For this review, take the finished solid that the model builds, in its own axes (mm). Give positions to 0.01 mm unless a question says otherwise; leave off trailing zeros. Write each loop counter-clockwise with the first axis right and the second up, starting at its lowest first coordinate (ties: lowest second). Pieces come first, ordered by that corner, then holes.
Q1. We need section A-A (z = 0). Write out the cut boundary in (x, y) (3 decimals).
Q2. Insertion check: P1, Ø8.5, axis at x = -29.48, z = 29.48, coming from the -Y side. The pin has a flat end and moves straight along its axis. Give the tip position at first contact, or say it passes through.
Q3. Mouldability with a two-part tool opening along Z and no side actions: class faces 1 (the cylindrical face through (-32.001, 87.072, 31.413)), 2 (the cylindrical face through (-26.454, 87.072, -30.436)), 3 (the flat face through (-35.687, 87, 0)), 4 (the flat face through (0, 87, 35.687)) as released by +Z, released by -Z, zero draft, split by the parting line, or undercut.
Q4. We need section C-C (y = 88.1). Write out the cut boundary in (x, z) (3 decimals), then the cut area to 3 significant figures.
Q5. We need section D-D (x = 29). Write out the cut boundary in (y, z).
Q6. For line 1 (X direction, y = 86.4, z = 31); line 2 (Z direction, x = 0, y = 86.75) (3 decimals), list the stretches that pass through material, from the lowest coordinate up.
Q7. We need section B-B (x = 0). Write out the cut boundary in (y, z) (3 decimals), then the cut area to 3 significant figures.
```python
from build123d import *

# Parameters (mm, degrees)
SKETCH3_W            = 71.374
SKETCH3_H            = 71.374
BOSS_EXTRUDE1_DEPTH  = 88.9508
SHELL1_T             = 5.08
CUT_EXTRUDE1_REACH   = 7.08
SKETCH4_R            = 8.255
SKETCH15_OUTSIDE_W   = 100.282
SKETCH15_OUTSIDE_H   = 117.859
SKETCH15_OUTSIDE_W_2 = 71.374
SKETCH15_OUTSIDE_H_2 = 3.81
CUT_EXTRUDE14_DEPTH  = 72.374
CUT_EXTRUDE15_START  = 88.9508
SKETCH20_R           = 3.175
CUT_EXTRUDE15_DEPTH  = 89.9508
SKETCH6_W            = 71.374
SKETCH6_H            = 5.08
CUT_EXTRUDE3_DEPTH   = 5.08


with BuildPart() as part:
    # Sketch3 → Boss-Extrude1 (new body)
    with BuildSketch(Plane(origin=(0, 0, 0), x_dir=(1, 0, 0), z_dir=(0, 1, 0))):
        Rectangle(SKETCH3_W, SKETCH3_H)
    extrude(amount=BOSS_EXTRUDE1_DEPTH)

    # Shell1 (no face opened: a closed hollow body)
    add(offset(amount=-SHELL1_T, mode=Mode.PRIVATE), mode=Mode.SUBTRACT)

    # Sketch4 → Cut-Extrude1 (cut, up to next)
    with BuildSketch(Plane(origin=(0, 83.8708, 0), x_dir=(-1, 0, 0), z_dir=(0, -1, 0)), mode=Mode.PRIVATE) as cut_extrude1_sk1:
        Circle(SKETCH4_R)
    cut_extrude1_tool1 = extrude(cut_extrude1_sk1.sketch, amount=-CUT_EXTRUDE1_REACH, mode=Mode.PRIVATE) & part.part
    add(cut_extrude1_tool1.solids().sort_by_distance((0, 83.8708, 0))[0], mode=Mode.SUBTRACT)

    # Sketch15 outside → Cut-Extrude14 (cut, through all)
    with BuildSketch(Plane.XY.offset(35.687)):
        with Locations((0, 44.4755)):
            Rectangle(SKETCH15_OUTSIDE_W, SKETCH15_OUTSIDE_H)
        with Locations((0, 87.0458)):
            Rectangle(SKETCH15_OUTSIDE_W_2, SKETCH15_OUTSIDE_H_2, mode=Mode.SUBTRACT)
    extrude(amount=-CUT_EXTRUDE14_DEPTH, mode=Mode.SUBTRACT)

    # Sketch20 → Cut-Extrude15 (cut, through all)
    with BuildSketch(Plane(origin=(0, 0, 0), x_dir=(1, 0, 0), z_dir=(0, 1, 0)).offset(CUT_EXTRUDE15_START)):
        with Locations((-29.482513587, 29.482513587)):
            Circle(SKETCH20_R)
        with Locations((29.484795022, -29.484795022)):
            Circle(SKETCH20_R)
        with Locations((-29.48121109, -29.48121109)):
            Circle(SKETCH20_R)
        with Locations((29.484795022, 29.484795022)):
            Circle(SKETCH20_R)
    extrude(amount=-CUT_EXTRUDE15_DEPTH, mode=Mode.SUBTRACT)

    # Sketch6 → Cut-Extrude3 (cut)
    with BuildSketch(Plane(origin=(0, 0, 30.607), x_dir=(-1, 0, 0), z_dir=(0, 0, -1))):
        with Locations((0, 2.54)):
            Rectangle(SKETCH6_W, SKETCH6_H)
    extrude(amount=-CUT_EXTRUDE3_DEPTH, mode=Mode.SUBTRACT)


solid = part.part
```
Computed:
1. outline: (-35.687, 85.141) - (-8.255, 85.141) - (-8.255, 88.951) - (-35.687, 88.951) - close; (8.255, 85.141) - (35.687, 85.141) - (35.687, 88.951) - (8.255, 88.951) - close
2. P1: stops at y = 85.14
3. face 1: undercut
3. face 2: undercut
3. face 3: zero draft
3. face 4: released by +Z
4. outline: (-35.687, -35.687) - (35.687, -35.687) - (35.687, 35.687) - (-35.687, 35.687) - close; hole circle Ø6.35 at (-29.483, -29.483); hole circle Ø6.35 at (-29.481, 29.481); hole circle Ø16.51 at (0, 0); hole circle Ø6.35 at (29.485, -29.485); hole circle Ø6.35 at (29.485, 29.485)
4. area: 4,750 mm2
5. outline: (85.14, -35.69) - (88.95, -35.69) - (88.95, -32.62) - (85.14, -32.62) - close; (85.14, -26.35) - (88.95, -26.35) - (88.95, 26.35) - (85.14, 26.35) - close; (85.14, 32.62) - (88.95, 32.62) - (88.95, 35.69) - (85.14, 35.69) - close
6. line 1: x = -35.69 to -32.27, -26.69 to 26.69, 32.27 to 35.69
6. line 2: z = -35.687 to -8.255, 8.255 to 35.687
7. outline: (85.141, -35.687) - (88.951, -35.687) - (88.951, -8.255) - (85.141, -8.255) - close; (85.141, 8.255) - (88.951, 8.255) - (88.951, 35.687) - (85.141, 35.687) - close
7. area: 209 mm2
